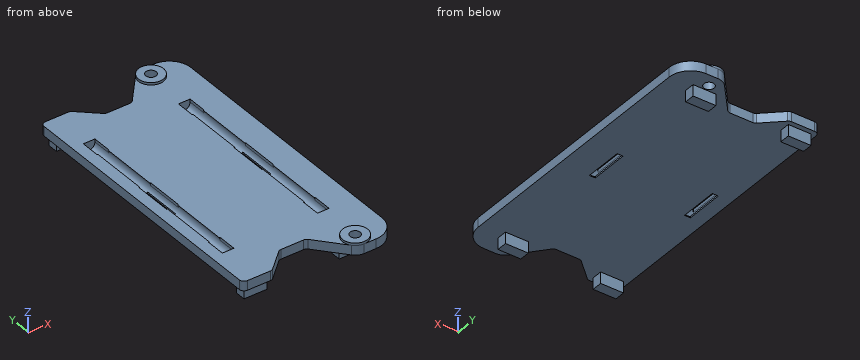
from build123d import *

# Parameters (mm, degrees)
SKETCH3_R           = 1.373
DOWEL_BODIES_DEPTH  = 13
BOSS_EXTRUDE3_DEPTH = 2.54
SKETCH5_W           = 6.096
SKETCH5_H           = 2.746000096
BOSS_EXTRUDE4_DEPTH = 3
SKETCH6_R           = 3.33375
SKETCH6_R_2         = 1.373
BOSS_EXTRUDE7_DEPTH = 0.635
SKETCH8_R           = 1.55
CUT_EXTRUDE1_DEPTH  = 25.4
CUT_EXTRUDE2_REACH  = 199.349
SKETCH9_W           = 1.5875
SKETCH9_H           = 10.16
CUT_EXTRUDE3_START  = -0.788
SKETCH10_W          = 3.1
SKETCH10_H          = 5.08
SKETCH10_H_2        = 10.16
CUT_EXTRUDE3_DEPTH  = 0.788
LPATTERN1_COUNT     = 2
LPATTERN1_PITCH     = 25.4


with BuildPart() as part:
    # Sketch3 → Dowel Bodies (new body)
    with BuildSketch(Plane.XY):
        with Locations(Location((184.15, 37.30625, 0), (0, 0, 180))):
            Circle(SKETCH3_R)
    extrude(amount=DOWEL_BODIES_DEPTH)


with BuildPart() as body_2:
    # Sketch4 → Boss-Extrude3 (new body)
    with BuildSketch(Plane.XY):
        with BuildLine():
            Line((168.402, 31.75), (174.498, 31.75))
            ThreePointArc((174.498, 31.75), (174.987232511, 31.857499863), (175.386332323, 32.160194447))
            Line((175.386332323, 32.160194447), (181.612315337, 39.468204119))
            ThreePointArc((181.612315337, 39.468204119), (182.752417351, 40.332906869), (184.15, 40.64))
            Line((184.15, 40.64), (187.325, 40.64))
            ThreePointArc((187.325, 40.64), (191.366115254, 38.966115254), (193.04, 34.925))
            Line((193.04, 34.925), (193.04, 0))
            Line((193.04, 0), (154.432, 0))
            Line((154.432, 0), (154.432, 35.663000048))
            ThreePointArc((154.432, 35.663000048), (154.803974388, 36.56102566), (155.702, 36.933000048))
            Line((155.702, 36.933000048), (161.798, 36.933000048))
            ThreePointArc((161.798, 36.933000048), (162.258293304, 36.846651211), (162.655994809, 36.599346622))
            Line((162.655994809, 36.599346622), (167.613590629, 32.056593332))
            ThreePointArc((167.613590629, 32.056593332), (167.979037588, 31.829345739), (168.402, 31.75))
        make_face()
    extrude(amount=BOSS_EXTRUDE3_DEPTH)

    # Combine1: cut part
    add(part.part, mode=Mode.SUBTRACT)

    # Sketch5 → Boss-Extrude4 (add)
    with BuildSketch(Plane(origin=(0, 0, 0), x_dir=(-1, 0, 0), z_dir=(0, 0, -1))):
        with Locations((-184.15, 34.29)):
            Rectangle(SKETCH5_W, SKETCH5_H)
        with Locations((-158.75, 34.29)):
            Rectangle(SKETCH5_W, SKETCH5_H)
    extrude(amount=BOSS_EXTRUDE4_DEPTH)

    # Sketch6 → Boss-Extrude7 (add)
    with BuildSketch(Plane.XY.offset(2.54)):
        with Locations(Location((184.15, 37.30625, 0), (0, 0, 139.571007131))):
            Circle(SKETCH6_R)
        with Locations(Location((184.15, 37.30625, 0), (0, 0, 180))):
            Circle(SKETCH6_R_2, mode=Mode.SUBTRACT)
    extrude(amount=BOSS_EXTRUDE7_DEPTH)

    # Mirror3: body 2 across plane


with BuildPart() as body_2_1:
    add(body_2.part)
    add(body_2.part.mirror(Plane.ZX))

    # Sketch8 → Cut-Extrude1 (cut, symmetric)
    with BuildSketch(Plane(origin=(0, 0, 0), x_dir=(1, 0, 0), z_dir=(0, 1, 0))):
        with Locations((158.951107585, -1.752)):
            Circle(SKETCH8_R)
    cut_extrude1 = extrude(amount=CUT_EXTRUDE1_DEPTH, both=True, mode=Mode.SUBTRACT)

    # Sketch9 → Cut-Extrude2 (cut, up to next)
    with BuildSketch(Plane.XY.offset(2.54), mode=Mode.PRIVATE) as cut_extrude2_sk1:
        with Locations((158.951107585, 0)):
            Rectangle(SKETCH9_W, SKETCH9_H)
    cut_extrude2_tool1 = extrude(cut_extrude2_sk1.sketch, amount=-CUT_EXTRUDE2_REACH, mode=Mode.PRIVATE) & body_2_1.part
    cut_extrude2 = cut_extrude2_tool1.solids().sort_by_distance((158.951108, 0, 2.54))[0]
    add(cut_extrude2, mode=Mode.SUBTRACT)

    # Sketch10 → Cut-Extrude3 (cut)
    with BuildSketch(Plane.XY.offset(2.54).offset(CUT_EXTRUDE3_START)):
        with Locations((158.951107585, 22.86)):
            Rectangle(SKETCH10_W, SKETCH10_H)
        with Locations((158.951107585, 0)):
            Rectangle(SKETCH10_W, SKETCH10_H_2)
        with Locations((158.951107585, -22.86)):
            Rectangle(SKETCH10_W, SKETCH10_H)
    cut_extrude3 = extrude(amount=CUT_EXTRUDE3_DEPTH, mode=Mode.SUBTRACT)

    # LPattern1: Cut-Extrude1, Cut-Extrude2, Cut-Extrude3 ×2
    with Locations(*[(i * LPATTERN1_PITCH, 0, 0) for i in range(1, LPATTERN1_COUNT)]):
        add(cut_extrude1, mode=Mode.SUBTRACT)
        add(cut_extrude2, mode=Mode.SUBTRACT)
        add(cut_extrude3, mode=Mode.SUBTRACT)


solid = body_2_1.part
Here's how the part is built. I have some questions about the finished solid (model axes, mm). Round coordinates to 2 decimals unless told otherwise and drop trailing zeros. Loops run counter-clockwise (first coordinate to the right, second up) from the corner with the lowest first, then second, coordinate; pieces in that order, holes last. Notation, with made-up numbers: (32.25, 4) - (60.25, 4) arc R32 ccw to (60.25, 33) - close; hole circle Ø11 at (-36.75, 33). An arc over 180 degrees is marked (long way). One line per question, with ' | ' between items. Start each with the question number.
Q1. I want a section at A-A (z = -1). Write out the boundary of the cut face in (x, y).
Q2. Will these pins go through, and if not, where does the flat tip stop? pin 1 (0.8 mm diameter, centred on x = 159.5, z = 1.5, fed in from -Y); pin 2 (8 mm diameter, centred on x = 188.5, y = -2, fed in from +Z); pin 3 (0.8 mm diameter, centred on x = 159, z = 0.5, fed in from +Y).
Q3. I want a section at B-B (y = -9.5). Write out the boundary of the cut face in (x, z), then the cut area to 3 significant figures.
Q4. Please list where these lines run through material, in increasing order: line 1 (Y direction, x = 184.15, z = 1.85); line 2 (Y direction, x = 160.5, z = -0.25); line 3 (X direction, y = 34, z = -1.25). Write a range as [from, to].
Q5. I want a section at C-C (x = 179.5). Write out the boundary of the cut face in (y, z), then the cut area to 3 significant figures.
Response values:
1) outline: (155.7, -35.66) - (161.8, -35.66) - (161.8, -32.92) - (155.7, -32.92) - close; (155.7, 32.92) - (161.8, 32.92) - (161.8, 35.66) - (155.7, 35.66) - close; (181.1, -35.66) - (187.2, -35.66) - (187.2, -32.92) - (181.1, -32.92) - close; (181.1, 32.92) - (187.2, 32.92) - (187.2, 35.66) - (181.1, 35.66) - close
2) pin 1: stops at y = -36.93 | pin 2: stops at z = 2.54 | pin 3: stops at y = 36.93
3) outline: (154.43, 0) - (193.04, 0) - (193.04, 2.54) - (185.69, 2.54) arc R1.55 cw (long way) to (183.02, 2.54) - (160.29, 2.54) arc R1.55 cw (long way) to (157.62, 2.54) - (154.43, 2.54) - close | area: 85.9 mm²
4) line 1: y = [-40.64, -38.68], [-35.93, -25.4], [25.4, 35.93], [38.68, 40.64] | line 2: y = [-35.66, -32.92], [32.92, 35.66] | line 3: x = [155.7, 161.8], [181.1, 187.2]
5) outline: (-36.99, 0) - (36.99, 0) - (36.99, 2.54) - (-36.99, 2.54) - close | area: 188 mm²
